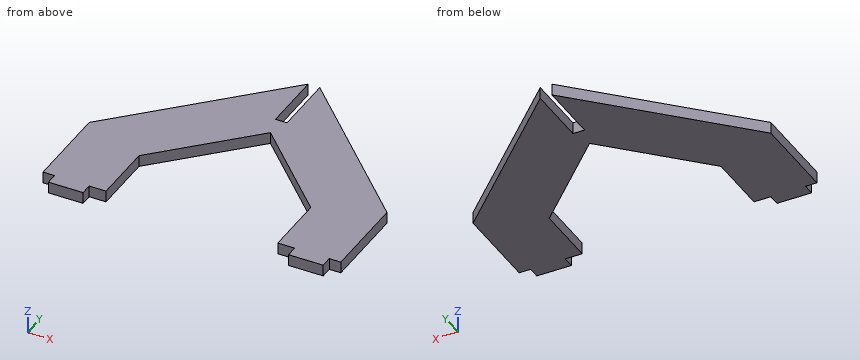
from build123d import *

# Parameters (mm, degrees)
BOSS_EXTRUDE1_DEPTH = 5
CUT_EXTRUDE1_DEPTH  = 10
SKETCH3_W           = 102.016100564
SKETCH3_H           = 114.3636127
CUT_EXTRUDE2_DEPTH  = 10
SKETCH4_W           = 42.096187012
SKETCH4_H           = 80.761359859
CUT_EXTRUDE3_DEPTH  = 10
SKETCH5_W           = 5
SKETCH5_H           = 58.521368684
CUT_EXTRUDE4_DEPTH  = 10


with BuildPart() as part:
    # Sketch1 → Boss-Extrude1 (new body)
    with BuildSketch(Plane.XY):
        Polygon((34.65186026, 42.723894515), (99.138982873, 107.211017127), (200, 6.35), (185, 6.35), (185, 0), (170, 0), (170, 6.35), (165, 6.35), (100.675, 70.675), (61.950419081, 31.950419081), (61.950419081, 5), (54.65186026, 5), (54.65186026, 0), (39.65186026, 0), (39.65186026, 5), (34.65186026, 5), align=None)
    boss_extrude1 = extrude(amount=BOSS_EXTRUDE1_DEPTH)

    # Sketch2 → Cut-Extrude1 (cut)
    with BuildSketch(Plane.XY.offset(5)):
        Polygon((96.638982873, 104.711017127), (96.638982873, 80.711017127), (101.638982873, 80.711017127), (101.638982873, 104.711017127), (99.138982873, 107.211017127), align=None)
    extrude(amount=-CUT_EXTRUDE1_DEPTH, mode=Mode.SUBTRACT)

    # Sketch3 → Cut-Extrude2 (cut)
    with BuildSketch(Plane.XY.offset(5)):
        with Locations((150.147033155, 51.840357155)):
            Rectangle(SKETCH3_W, SKETCH3_H)
    extrude(amount=-CUT_EXTRUDE2_DEPTH, mode=Mode.SUBTRACT)

    # Mirror1: Boss-Extrude1 across plane
    add(boss_extrude1.mirror(Plane(origin=(99.138982873, 109.022163505, -5), x_dir=(0, 0, 1), z_dir=(-1, 0, 0))))

    # Sketch4 → Cut-Extrude3 (cut)
    with BuildSketch(Plane(origin=(0, 0, 0), x_dir=(-1, 0, 0), z_dir=(0, 0, -1))):
        with Locations((-13.603766754, 32.73650171)):
            Rectangle(SKETCH4_W, SKETCH4_H)
    extrude(amount=-CUT_EXTRUDE3_DEPTH, mode=Mode.SUBTRACT)

    # Sketch5 → Cut-Extrude4 (cut)
    with BuildSketch(Plane(origin=(0, 0, 0), x_dir=(-1, 0, 0), z_dir=(0, 0, -1))):
        with Locations((-99.138982873, 107.211017127)):
            Rectangle(SKETCH5_W, SKETCH5_H)
    extrude(amount=-CUT_EXTRUDE4_DEPTH, mode=Mode.SUBTRACT)


solid = part.part
Here's how the part is built. I have some questions about the finished solid (model axes, mm). Round coordinates to 2 decimals unless told otherwise and drop trailing zeros. Write each loop counter-clockwise with the first axis right and the second up, starting at its lowest first coordinate (ties: lowest second). Pieces come first, ordered by that corner, then holes.
1. I need wall thicknesses on L1, parallel to X at y = 20, z = 4.05; L2, parallel to X at y = 45, z = 1; L3, parallel to Y at x = 129, z = 0.4. Which ranges of each line are inside material? Lowest first, please.
2. Suppose I cut it at D-D (y = 92). List the corners of the cut face in (x, z) for me.
3. Suppose I cut it at A-A (y = 28). List the corners of the cut face in (x, z) for me.
4. Suppose I cut it at B-B (z = 3.35). List the corners of the cut face in (x, y) for me, and give its area (3 significant figures).
5. Will these pins go through, and if not, where does the flat tip stop? pin 1 Ø1.5 at (x, z) = (100, 1.5) entering from +Y; pin 2 Ø2.5 at (y, z) = (1.5, 3) entering from -X; pin 3 Ø1.5 at (y, z) = (3, 1.5) entering from +X.
6. Suppose I cut it at C-C (x = 152). List the corners of the cut face in (y, z) for me, and give its area (3 significant figures).
Answer sheet:
1. L1: x = 34.65 to 61.95, 136.33 to 163.63
1. L2: x = 36.93 to 75, 123.28 to 161.35
1. L3: y = 39.28 to 77.35
2. outline: (83.93, 0) - (96.64, 0) - (96.64, 5) - (83.93, 5) - close; (101.64, 0) - (114.35, 0) - (114.35, 5) - (101.64, 5) - close
3. outline: (34.65, 0) - (61.95, 0) - (61.95, 5) - (34.65, 5) - close; (136.33, 0) - (163.63, 0) - (163.63, 5) - (136.33, 5) - close
4. outline: (34.65, 5) - (39.65, 5) - (39.65, 0) - (54.65, 0) - (54.65, 5) - (61.95, 5) - (61.95, 31.95) - (99.14, 69.14) - (136.33, 31.95) - (136.33, 5) - (143.63, 5) - (143.63, 0) - (158.63, 0) - (158.63, 5) - (163.63, 5) - (163.63, 42.72) - (101.64, 104.71) - (101.64, 77.95) - (96.64, 77.95) - (96.64, 104.71) - (34.65, 42.72) - close
4. area: 5,650 mm2
5. pin 1: stops at y = 77.95
5. pin 2: stops at x = 39.65
5. pin 3: stops at x = 158.63
6. outline: (0, 0) - (54.35, 0) - (54.35, 5) - (0, 5) - close
6. area: 272 mm2
